```python
from build123d import *

# Parameters (mm, degrees)
F0_W     = 99.06
F0_H     = 99.06
F1_DEPTH = 35.56
F2_R     = 12.7
F3_W     = 25.4
F3_H     = 12.7
F4_DEPTH = 2.54


with BuildPart() as f1:
    # F0 (on Top) → F1 (new body)
    with BuildSketch(Plane.XY):
        Rectangle(F0_W, F0_H)
    extrude(amount=F1_DEPTH)

    # F2
    f2_edges = [f1.edges().sort_by_distance(p)[0] for p in [
        (49.53, -49.53, 17.78),
        (49.53, 49.53, 17.78),
        (-49.53, -49.53, 17.78),
        (-49.53, 49.53, 17.78),
    ]]
    fillet(f2_edges, radius=F2_R)

    # F3 (on face) → F4 (cut)
    with BuildSketch(Plane(origin=(0, 49.53, 0), x_dir=(-1, 0, 0), z_dir=(0, 1, 0))):
        with Locations((0, 17.78)):
            Rectangle(F3_W, F3_H)
    extrude(amount=-F4_DEPTH, mode=Mode.SUBTRACT)


solid = f1.part
```
CAD build for the part. Positions are in the model's coordinates, mm. A direction names the side the tool comes from. Round coordinates to 2 decimals unless told otherwise and drop trailing zeros. Order: outer loops, then holes, each group sorted by start corner. A loop starts at its lowest first (then second) coordinate and runs counter-clockwise, first axis right, second up. Notation, with made-up numbers: (54.5, 34) -> (82.5, 34) arc R14 cw to (82.5, 40) -> close; hole circle Ø3 at (-10.5, -7.5). An arc over 180 degrees is marked (long way). Write item = value, one per line.
(1) Flat gauge pins, fed straight in: P1, Ø2, axis at x = -1.5, y = 48.5, coming from the -Z side; P2, Ø2, axis at y = 48, z = 15.5, coming from the +X side; P3, Ø6.5, axis at x = -3, z = 19, coming from the +Y side; P4, Ø3, axis at y = 47.5, z = 19, coming from the -X side. Where does each tip first touch, or does it go through?
Answers follow:
P1 = 0
P2 = 44.44
P3 = 46.99
P4 = -45.62
(2) 3-axis set-ups, long thin cutter, end or side, ignore diameter. For faces 1 (the cylindrical face through (-45.91, -45.71, 18.03)), 2 (the flat face through (0, 46.99, 18)): which of +Z, -Z, +X, -X, +Y, -Y reach the whole face in a straight line?
Answers follow:
face_1 = +Z, -Z, -X, -Y
face_2 = +Y
(3) Drill centre lines: L1, parallel to Y at x = -9, z = 21.5; L2, parallel to X at y = 42.5, z = 30; L3, parallel to Y at x = -44.5, z = 6. Where is each one in solid material? Low to high.
Answers follow:
L1 = -49.53 to 46.99
L2 = -48.19 to 48.19
L3 = -46.95 to 46.95
(4) Pull direction X, two halves, no side cores. Call faces 3 (the cylindrical face through (-45.91, 45.71, 18.03)), 4 (the flat face through (49.53, -1, 18)), 5 (the flat face through (0, 48, 11.43)): +X half, -X half, draft (parallel to the pull), parting line (faces both ways), or undercut.
Answers follow:
face_3 = -X half
face_4 = +X half
face_5 = undercut
(5) Cut at A-A (z = 13). Write the cut outline in (x, y).
Answers follow:
outline = (-49.53, -36.83) arc R12.7 ccw to (-36.83, -49.53) -> (36.83, -49.53) arc R12.7 ccw to (49.53, -36.83) -> (49.53, 36.83) arc R12.7 ccw to (36.83, 49.53) -> (12.7, 49.53) -> (12.7, 46.99) -> (-12.7, 46.99) -> (-12.7, 49.53) -> (-36.83, 49.53) arc R12.7 ccw to (-49.53, 36.83) -> close
